Check sheet for the modelled part. Datum: model origin and axes. Units: mm. Give positions to 0.01 mm unless a question says otherwise; leave off trailing zeros. Write each loop counter-clockwise with the first axis right and the second up, starting at its lowest first coordinate (ties: lowest second). Pieces come first, ordered by that corner, then holes. Notation, with made-up numbers: (57, -13) -> (104, -13) arc R23 cw to (104, 4) -> close; hole circle Ø2 at (7, 35). An arc over 180 degrees is marked (long way). Return JSON: item names as keys, results as strings.
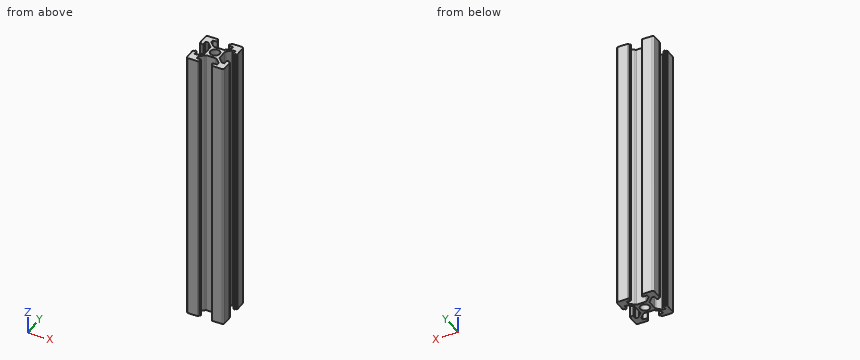
from build123d import *

# Parameters (mm, degrees)
SKETCH2_R           = 2.5
BOSS_EXTRUDE1_DEPTH = 150


with BuildPart() as part:
    # Sketch2 → Boss-Extrude1 (new body)
    with BuildSketch(Plane.XY):
        with BuildLine():
            ThreePointArc((4, 10), (3.646446609, 9.853553391), (3.5, 9.5))
            Line((3.5, 9.5), (3.5, 9.25))
            ThreePointArc((3.5, 9.25), (3.426776695, 9.073223305), (3.25, 9))
            Line((3.25, 9), (3.2, 9))
            ThreePointArc((3.2, 9), (3.058578644, 8.941421356), (3, 8.8))
            Line((3, 8.8), (3, 8.5))
            ThreePointArc((3, 8.5), (3.146446609, 8.146446609), (3.5, 8))
            Line((3.5, 8), (5.5, 8))
            Line((5.5, 8), (5.5, 6.560660172))
            Line((5.5, 6.560660172), (3.107233047, 4.167893219))
            ThreePointArc((3.107233047, 4.167893219), (2.782809698, 3.951120467), (2.400126266, 3.875))
            Line((2.400126266, 3.875), (0, 3.875))
            Line((0, 3.875), (-2.400126266, 3.875))
            ThreePointArc((-2.400126266, 3.875), (-2.782809698, 3.951120467), (-3.107233047, 4.167893219))
            Line((-3.107233047, 4.167893219), (-5.5, 6.560660172))
            Line((-5.5, 6.560660172), (-5.5, 8))
            Line((-5.5, 8), (-3.5, 8))
            ThreePointArc((-3.5, 8), (-3.146446609, 8.146446609), (-3, 8.5))
            Line((-3, 8.5), (-3, 8.8))
            ThreePointArc((-3, 8.8), (-3.058578644, 8.941421356), (-3.2, 9))
            Line((-3.2, 9), (-3.25, 9))
            ThreePointArc((-3.25, 9), (-3.426776695, 9.073223305), (-3.5, 9.25))
            Line((-3.5, 9.25), (-3.5, 9.5))
            ThreePointArc((-3.5, 9.5), (-3.646446609, 9.853553391), (-4, 10))
            Line((-4, 10), (-9, 10))
            ThreePointArc((-9, 10), (-9.707106781, 9.707106781), (-10, 9))
            Line((-10, 9), (-10, 4))
            ThreePointArc((-10, 4), (-9.853553391, 3.646446609), (-9.5, 3.5))
            Line((-9.5, 3.5), (-9.25, 3.5))
            ThreePointArc((-9.25, 3.5), (-9.073223305, 3.426776695), (-9, 3.25))
            Line((-9, 3.25), (-9, 3.2))
            ThreePointArc((-9, 3.2), (-8.941421356, 3.058578644), (-8.8, 3))
            Line((-8.8, 3), (-8.5, 3))
            ThreePointArc((-8.5, 3), (-8.146446609, 3.146446609), (-8, 3.5))
            Line((-8, 3.5), (-8, 5.5))
            Line((-8, 5.5), (-6.560660172, 5.5))
            Line((-6.560660172, 5.5), (-4.167893219, 3.107233047))
            ThreePointArc((-4.167893219, 3.107233047), (-3.951120467, 2.782809698), (-3.875, 2.400126266))
            Line((-3.875, 2.400126266), (-3.875, 0))
            Line((-3.875, 0), (-3.875, -2.400126266))
            ThreePointArc((-3.875, -2.400126266), (-3.951120467, -2.782809698), (-4.167893219, -3.107233047))
            Line((-4.167893219, -3.107233047), (-6.560660172, -5.5))
            Line((-6.560660172, -5.5), (-8, -5.5))
            Line((-8, -5.5), (-8, -3.5))
            ThreePointArc((-8, -3.5), (-8.146446609, -3.146446609), (-8.5, -3))
            Line((-8.5, -3), (-8.8, -3))
            ThreePointArc((-8.8, -3), (-8.941421356, -3.058578644), (-9, -3.2))
            Line((-9, -3.2), (-9, -3.25))
            ThreePointArc((-9, -3.25), (-9.073223305, -3.426776695), (-9.25, -3.5))
            Line((-9.25, -3.5), (-9.5, -3.5))
            ThreePointArc((-9.5, -3.5), (-9.853553391, -3.646446609), (-10, -4))
            Line((-10, -4), (-10, -9))
            ThreePointArc((-10, -9), (-9.707106781, -9.707106781), (-9, -10))
            Line((-9, -10), (-4, -10))
            ThreePointArc((-4, -10), (-3.646446609, -9.853553391), (-3.5, -9.5))
            Line((-3.5, -9.5), (-3.5, -9.25))
            ThreePointArc((-3.5, -9.25), (-3.426776695, -9.073223305), (-3.25, -9))
            Line((-3.25, -9), (-3.2, -9))
            ThreePointArc((-3.2, -9), (-3.058578644, -8.941421356), (-3, -8.8))
            Line((-3, -8.8), (-3, -8.5))
            ThreePointArc((-3, -8.5), (-3.146446609, -8.146446609), (-3.5, -8))
            Line((-3.5, -8), (-5.5, -8))
            Line((-5.5, -8), (-5.5, -6.560660172))
            Line((-5.5, -6.560660172), (-3.107233047, -4.167893219))
            ThreePointArc((-3.107233047, -4.167893219), (-2.782809698, -3.951120467), (-2.400126266, -3.875))
            Line((-2.400126266, -3.875), (0, -3.875))
            Line((0, -3.875), (2.400126266, -3.875))
            ThreePointArc((2.400126266, -3.875), (2.782809698, -3.951120467), (3.107233047, -4.167893219))
            Line((3.107233047, -4.167893219), (5.5, -6.560660172))
            Line((5.5, -6.560660172), (5.5, -8))
            Line((5.5, -8), (3.5, -8))
            ThreePointArc((3.5, -8), (3.146446609, -8.146446609), (3, -8.5))
            Line((3, -8.5), (3, -8.8))
            ThreePointArc((3, -8.8), (3.058578644, -8.941421356), (3.2, -9))
            Line((3.2, -9), (3.25, -9))
            ThreePointArc((3.25, -9), (3.426776695, -9.073223305), (3.5, -9.25))
            Line((3.5, -9.25), (3.5, -9.5))
            ThreePointArc((3.5, -9.5), (3.646446609, -9.853553391), (4, -10))
            Line((4, -10), (9, -10))
            ThreePointArc((9, -10), (9.707106781, -9.707106781), (10, -9))
            Line((10, -9), (10, -4))
            ThreePointArc((10, -4), (9.853553391, -3.646446609), (9.5, -3.5))
            Line((9.5, -3.5), (9.25, -3.5))
            ThreePointArc((9.25, -3.5), (9.073223305, -3.426776695), (9, -3.25))
            Line((9, -3.25), (9, -3.2))
            ThreePointArc((9, -3.2), (8.941421356, -3.058578644), (8.8, -3))
            Line((8.8, -3), (8.5, -3))
            ThreePointArc((8.5, -3), (8.146446609, -3.146446609), (8, -3.5))
            Line((8, -3.5), (8, -5.5))
            Line((8, -5.5), (6.560660172, -5.5))
            Line((6.560660172, -5.5), (4.167893219, -3.107233047))
            ThreePointArc((4.167893219, -3.107233047), (3.951120467, -2.782809698), (3.875, -2.400126266))
            Line((3.875, -2.400126266), (3.875, 0))
            Line((3.875, 0), (3.875, 2.400126266))
            ThreePointArc((3.875, 2.400126266), (3.951120467, 2.782809698), (4.167893219, 3.107233047))
            Line((4.167893219, 3.107233047), (6.560660172, 5.5))
            Line((6.560660172, 5.5), (8, 5.5))
            Line((8, 5.5), (8, 3.5))
            ThreePointArc((8, 3.5), (8.146446609, 3.146446609), (8.5, 3))
            Line((8.5, 3), (8.8, 3))
            ThreePointArc((8.8, 3), (8.941421356, 3.058578644), (9, 3.2))
            Line((9, 3.2), (9, 3.25))
            ThreePointArc((9, 3.25), (9.073223305, 3.426776695), (9.25, 3.5))
            Line((9.25, 3.5), (9.5, 3.5))
            ThreePointArc((9.5, 3.5), (9.853553391, 3.646446609), (10, 4))
            Line((10, 4), (10, 9))
            ThreePointArc((10, 9), (9.707106781, 9.707106781), (9, 10))
            Line((9, 10), (4, 10))
        make_face()
        Circle(SKETCH2_R, mode=Mode.SUBTRACT)
    extrude(amount=BOSS_EXTRUDE1_DEPTH)


solid = part.part
(1) Cross-section at A-A on y = 0. Enter the section's corners in (x, z) (3 decimals), then the cut area to 4 significant figures.
Reply:
{"outline": "(-3.875, 0) -> (-2.5, 0) -> (-2.5, 150) -> (-3.875, 150) -> close; (2.5, 0) -> (3.875, 0) -> (3.875, 150) -> (2.5, 150) -> close", "area": "412.5 mm^2"}
(2) Depth check by flat-ended pin: pin 1 Ø5.5 at (y, z) = (0, 62) entering from -X; pin 2 Ø4 at (x, y) = (0.5, -7) entering from +Z; pin 3 Ø1 at (x, z) = (-1, 30) entering from -Y (3 decimals). Enter the tip coordinate at first touch or a pass-through.
Reply:
{"pin 1": "x = -3.94", "pin 2": "through", "pin 3": "y = -3.875"}
(3) Thickness scan on L1, parallel to Y at x = -0.25, z = 38 (3 decimals); L2, parallel to Y at x = 8.75, z = 94; L3, parallel to Y at x = -4, z = 79. Record the ranges inside material, lowest first.
Reply:
{"L1": "-3.875 to -2.487, 2.487 to 3.875", "L2": "-10 to -3, 3 to 10", "L3": "-10 to -8, -5.06 to -2.88, 2.88 to 5.06, 8 to 10"}
